Verification items for this drawing (mm, ordinates from the low corner). A direction names the side the tool comes from. Round coordinates to 2 decimals unless told otherwise and drop trailing zeros. Write each loop counter-clockwise with the first axis right and the second up, starting at its lowest first coordinate (ties: lowest second). Pieces come first, ordered by that corner, then holes. Notation, with made-up numbers: (71.25, 9) -> (89.25, 9) arc R14 cw to (89.25, 24) -> close; hole circle Ø4 at (-1.5, 27). An arc over 180 degrees is marked (long way). Return JSON: item names as keys, results as strings. Group by question number.
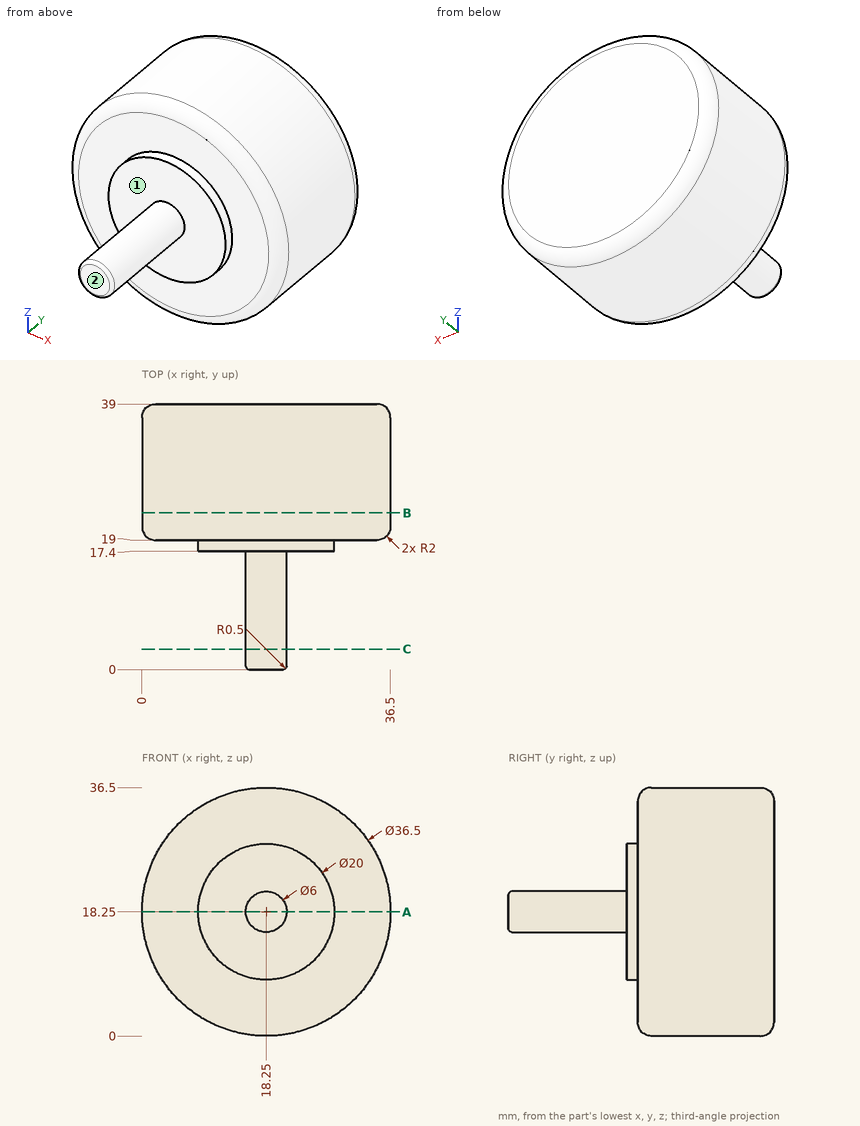
1) Sectioned sample at B-B on y = 23. Enter the section's corners in (x, z), and give its area (3 significant figures).
2) Sectioned sample at C-C on y = 3. Enter the section's corners in (x, z), and give its area (3 significant figures).
3) Sectioned sample at A-A on z = 18.25. Enter the section's corners in (x, y).
4) Go/stop test with flat-tipped pins: P1, Ø10, axis at x = 29, z = 25.5, coming from the -Y side; P2, Ø5, axis at y = 21.5, z = 31, coming from the +X side; P3, Ø1.5, axis at y = 20.5, z = 17, coming from the -X side. Record where each tip stops, or that it passes through.
5) Tool access check on the marked faces 1 and 2. Record the directions out of +Z, -Z, +X, -X, +Y, -Y that give a thin tool (end or side, any length) a straight path to the whole face; none if there is none.
6) Material ranges on probe 1 along Y at (x, z) = (26, 21.5); probe 2 along Y at (x, z) = (15.5, 28); probe 3 along Z at (x, y) = (35, 33.5), recorded low to high. Write a range as [from, to].
Evaluation:
{
 "1": {"outline": "circle Ø36.5 at (18.25, 18.25)", "area": "1,050 mm2"},
 "2": {"outline": "circle Ø6 at (18.25, 18.25)", "area": "28.3 mm2"},
 "3": {"outline": "(0, 21) arc R2 ccw to (2, 19) -> (8.25, 19) -> (8.25, 17.4) -> (15.25, 17.4) -> (15.25, 0.5) arc R0.5 ccw to (15.75, 0) -> (20.75, 0) arc R0.5 ccw to (21.25, 0.5) -> (21.25, 17.4) -> (28.25, 17.4) -> (28.25, 19) -> (34.5, 19) arc R2 ccw to (36.5, 21) -> (36.5, 37) arc R2 ccw to (34.5, 39) -> (2, 39) arc R2 ccw to (0, 37) -> close"},
 "4": {"P1": "stops at y = 17.4", "P2": "stops at x = 33.35", "P3": "stops at x = 0.01"},
 "5": {"face 1": "-Y", "face 2": "+Z, -Z, +X, -X, -Y"},
 "6": {"probe 1": "y = [17.4, 39]", "probe 2": "y = [19, 39]", "probe 3": "z = [11, 25.5]"}
}
